The drawing under review shows one solid part. Ordinate dimensions are in mm from its lowest x, y, z. A direction names the side the tool comes from. Give positions to 0.01 mm unless a question says otherwise; leave off trailing zeros. Order: outer loops, then holes, each group sorted by start corner. A loop starts at its lowest first (then second) coordinate and runs counter-clockwise, first axis right, second up. Notation, with made-up numbers: (-14, -19.75) - (12, -19.75) arc R29 ccw to (12, 11.25) - close; hole circle Ø4 at (57.25, 45). An arc over 180 degrees is marked (long way). Write item = value, one per line. Start each with the question number.
1. For P1, Ø12, axis at x = 17, z = 19.5, coming from the -Y side; P2, Ø12, axis at x = 12, z = 38.5, coming from the +Y side; P3, Ø6, axis at y = 2, z = 27.5, coming from the +X side, all flat-tipped, find the tip position at first contact; note any pin that passes through.
2. Machinability: for the marked faces 1 and 2, which of the approach directions +Z, -Z, +X, -X, +Y, -Y give a long, thin tool a straight path to every point of the face, cutting with its end or side? Answer none if there is none.
3. We need section C-C, the plane z = 25.5. Give the boundary of the cut face in (x, y).
4. Wall thickness on probe 1 along Y at (x, z) = (10.5, 1.65); probe 2 along Z at (x, y) = (17, 7.5); probe 3 along Z at (x, y) = (2, 4.75): over which ranges is each line inside the solid? List them lowest first.
5. We need section D-D, the plane y = 3. Give the boundary of the cut face in (x, z).
6. We need section A-A, the plane y = 10.5. Give the boundary of the cut face in (x, z).
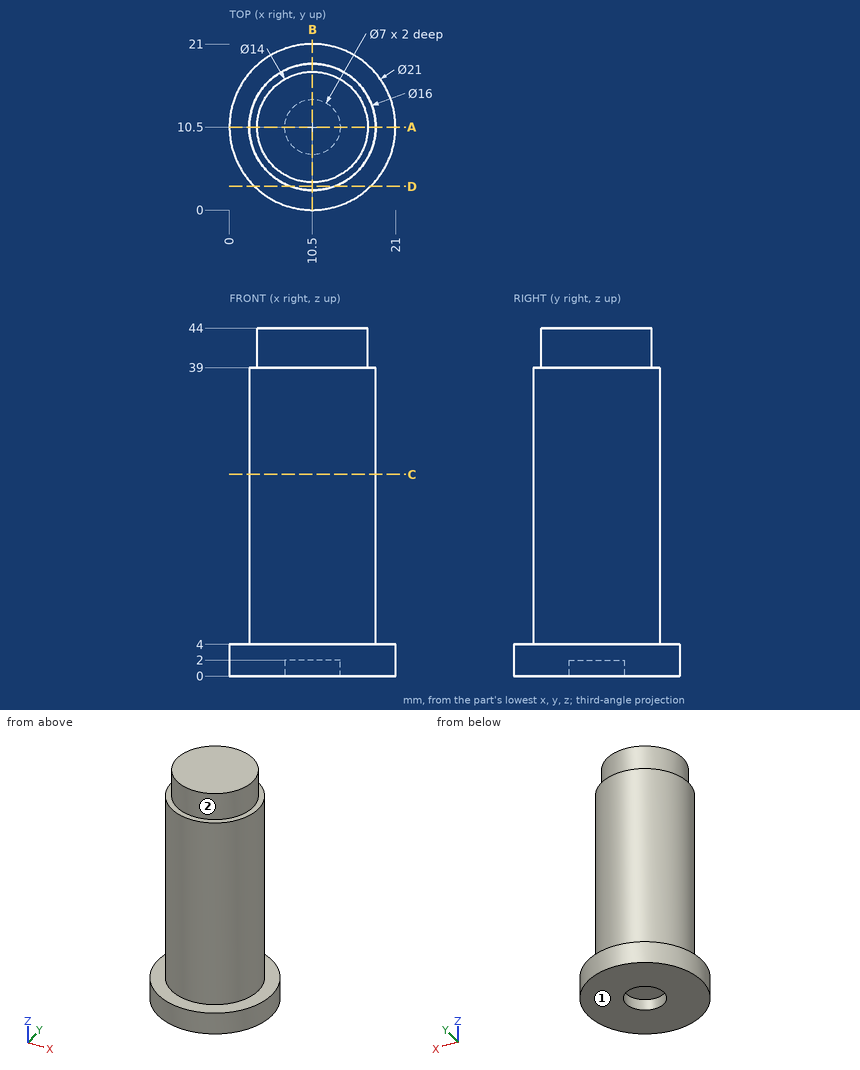
Model answer:
q1.P1 = 2.52
q1.P2 = 18.5
q1.P3 = 16.31
q2.face_1 = -Z, +X, -X, +Y, -Y
q2.face_2 = +Z
q3.outline = circle Ø16 at (10.5, 10.5)
q4.probe_1 = 0 to 7, 14 to 21
q4.probe_2 = 0 to 39
q4.probe_3 = 0 to 4
q5.outline = (3.15, 0) - (17.85, 0) - (17.85, 4) - (13.28, 4) - (13.28, 39) - (7.72, 39) - (7.72, 4) - (3.15, 4) - close
q6.outline = (0, 0) - (7, 0) - (7, 2) - (14, 2) - (14, 0) - (21, 0) - (21, 4) - (18.5, 4) - (18.5, 39) - (17.5, 39) - (17.5, 44) - (3.5, 44) - (3.5, 39) - (2.5, 39) - (2.5, 4) - (0, 4) - close
